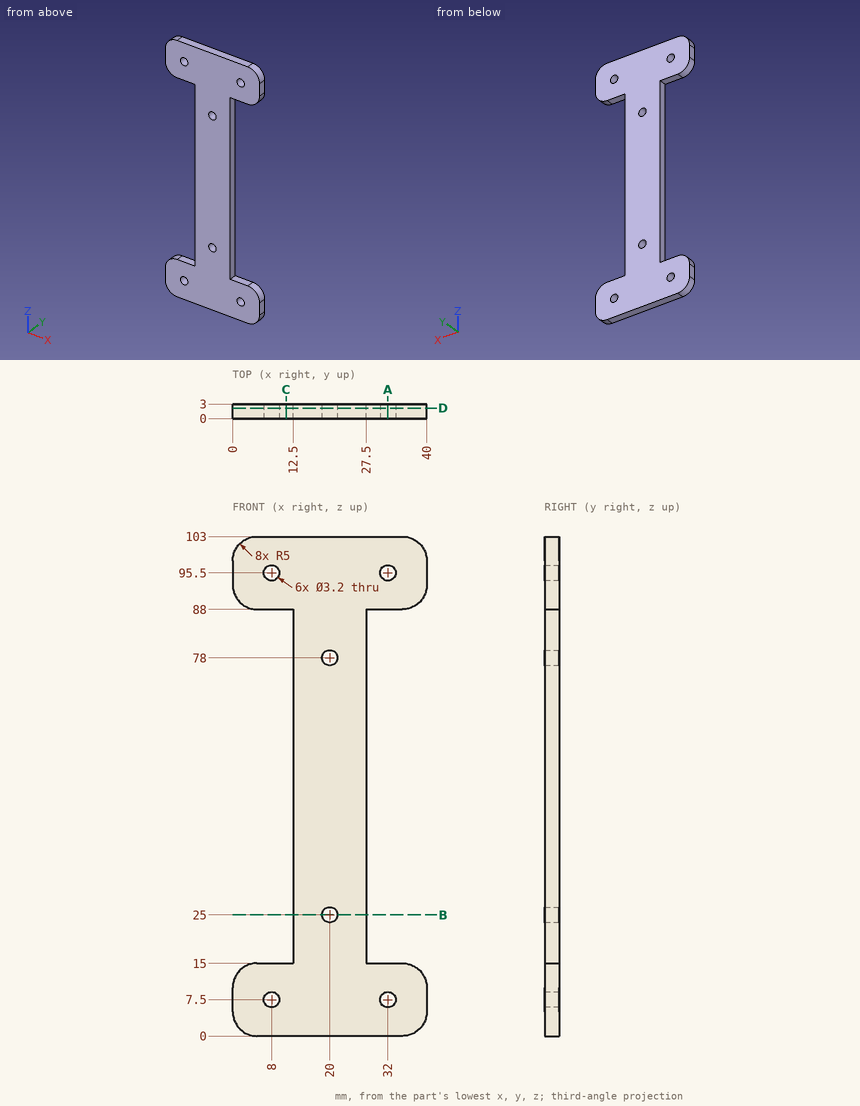
Job drawing, mm, ordinate dimensions from the low corner. One solid piece. Round coordinates to 2 decimals unless told otherwise and drop trailing zeros. Write each loop counter-clockwise with the first axis right and the second up, starting at its lowest first coordinate (ties: lowest second). Pieces come first, ordered by that corner, then holes.
1) Band-saw the part on A-A, the plane x = 32. List the corners of the cut face in (y, z), and give its area (3 significant figures).
2) Band-saw the part on D-D, the plane y = 2.15. List the corners of the cut face in (x, z), and give its area (3 significant figures).
3) Band-saw the part on B-B, the plane z = 25. List the corners of the cut face in (x, y), and give its area (3 significant figures).
4) Band-saw the part on C-C, the plane x = 11. List the corners of the cut face in (y, z).
5) Pin check, flat tips, straight feed: pin 1 (3 mm diameter, centred on x = 20, z = 78, fed in from +Y) (3 decimals); pin 2 (1.5 mm diameter, centred on y = 2, z = 35.5, fed in from -X). Stop position of each tip, or through.
6) Drill centre lines: probe 1 along X at (y, z) = (1.1, 7.5); probe 2 along X at (y, z) = (1.55, 25); probe 3 along Z at (x, y) = (11.5, 1.55). Where is each one in solid material? Low to high.
Ans:
1. outline: (0, 0) - (3, 0) - (3, 5.9) - (0, 5.9) - close; (0, 9.1) - (3, 9.1) - (3, 15) - (0, 15) - close; (0, 88) - (3, 88) - (3, 93.9) - (0, 93.9) - close; (0, 97.1) - (3, 97.1) - (3, 103) - (0, 103) - close
1. area: 70.8 mm2
2. outline: (0, 5) arc R5 ccw to (5, 0) - (35, 0) arc R5 ccw to (40, 5) - (40, 10) arc R5 ccw to (35, 15) - (27.5, 15) - (27.5, 88) - (35, 88) arc R5 ccw to (40, 93) - (40, 98) arc R5 ccw to (35, 103) - (5, 103) arc R5 ccw to (0, 98) - (0, 93) arc R5 ccw to (5, 88) - (12.5, 88) - (12.5, 15) - (5, 15) arc R5 ccw to (0, 10) - close; hole circle Ø3.2 at (8, 7.5); hole circle Ø3.2 at (8, 95.5); hole circle Ø3.2 at (20, 25); hole circle Ø3.2 at (20, 78); hole circle Ø3.2 at (32, 7.5); hole circle Ø3.2 at (32, 95.5)
2. area: 2,200 mm2
3. outline: (12.5, 0) - (18.4, 0) - (18.4, 3) - (12.5, 3) - close; (21.6, 0) - (27.5, 0) - (27.5, 3) - (21.6, 3) - close
3. area: 35.4 mm2
4. outline: (0, 0) - (3, 0) - (3, 15) - (0, 15) - close; (0, 88) - (3, 88) - (3, 103) - (0, 103) - close
5. pin 1: passes through
5. pin 2: stops at x = 12.5
6. probe 1: x = 0 to 6.4, 9.6 to 30.4, 33.6 to 40
6. probe 2: x = 12.5 to 18.4, 21.6 to 27.5
6. probe 3: z = 0 to 15, 88 to 103
